Print and shaded views of the part. All mm, measured from the part's lowest x, y and z. Round coordinates to 2 decimals unless told otherwise and drop trailing zeros. Order: outer loops, then holes, each group sorted by start corner. A loop starts at its lowest first (then second) coordinate and runs counter-clockwise, first axis right, second up. Notation, with made-up numbers: (-20.5, 55) -> (34.5, 55) arc R29 cw to (34.5, 86) -> close; hole circle Ø4 at (10.25, -1). An arc over 180 degrees is marked (long way). Answer as CSV lines item,"result".
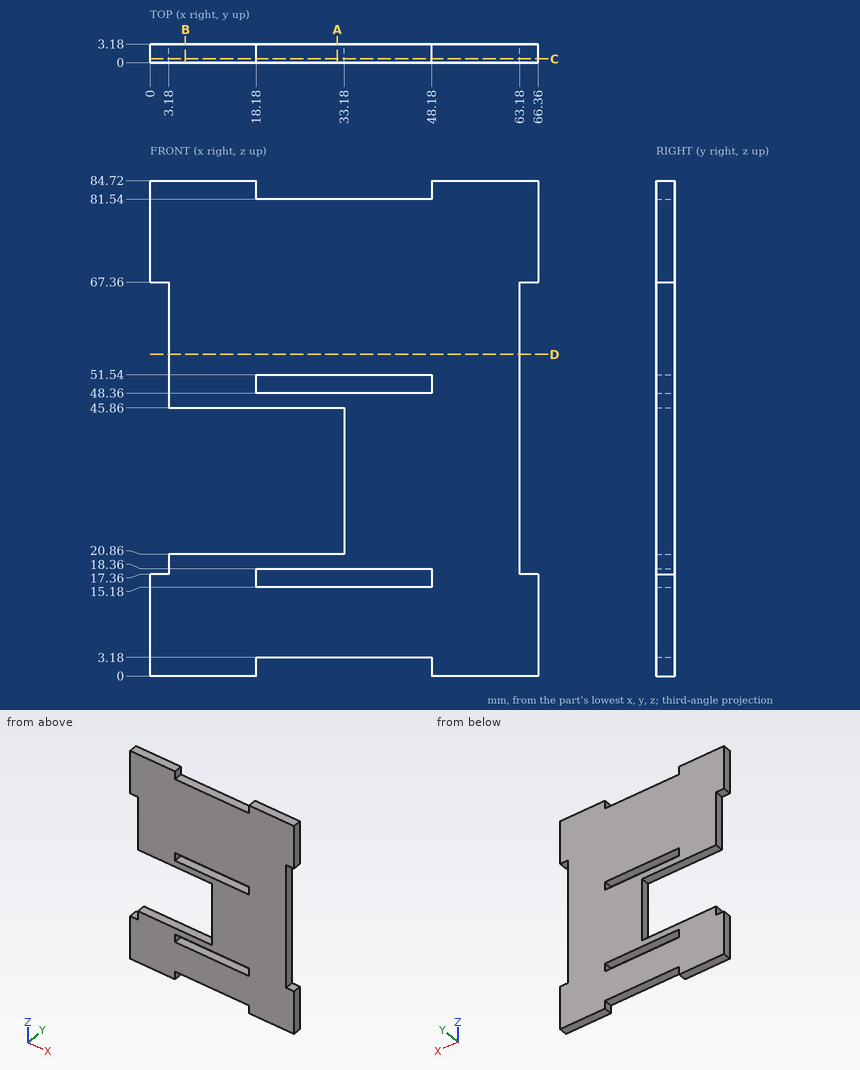
Q1. Saw through at C-C (y = 0.65). State how many separate pieces and enclosed holes the cut face has, plus the area to 3 significant figures.
Checks:
separate pieces,"1"
enclosed holes,"2"
area,"4,170 mm²"
Q2. Flat gauge pins, fed straight in: pin 1 (1.5 mm diameter, centred on y = 2, z = 48, fed in from -X); pin 2 (1.6 mm diameter, centred on x = 33, y = 1, fed in from -Z); pin 3 (1.6 mm diameter, centred on x = 20, y = 2, fed in from +Z). Where does each tip first touch, or does it go through?
Checks:
pin 1,"x = 3.18"
pin 2,"z = 3.18"
pin 3,"z = 81.54"
Q3. Saw through at A-A (x = 32). Write the cut outline in (y, z).
Checks:
outline,"(0, 3.18) -> (3.18, 3.18) -> (3.18, 15.18) -> (0, 15.18) -> close; (0, 18.36) -> (3.18, 18.36) -> (3.18, 20.86) -> (0, 20.86) -> close; (0, 45.86) -> (3.18, 45.86) -> (3.18, 48.36) -> (0, 48.36) -> close; (0, 51.54) -> (3.18, 51.54) -> (3.18, 81.54) -> (0, 81.54) -> close"
Q4. Wall check: L1, parallel to Z at x = 34, y = 1.9; L2, parallel to Z at x = 25, y = 1.1; L3, parallel to Z at x = 8, y = 2.25. Give the ranges that are in metal, low to high. Write a range as [from, to].
Checks:
L1,"[3.18, 15.18], [18.36, 48.36], [51.54, 81.54]"
L2,"[3.18, 15.18], [18.36, 20.86], [45.86, 48.36], [51.54, 81.54]"
L3,"[0, 20.86], [45.86, 84.72]"
Q5. Saw through at B-B (x = 6). Write the cut outline in (y, z).
Checks:
outline,"(0, 0) -> (3.18, 0) -> (3.18, 20.86) -> (0, 20.86) -> close; (0, 45.86) -> (3.18, 45.86) -> (3.18, 84.72) -> (0, 84.72) -> close"
Q6. Saw through at D-D (z = 55). Write the cut outline in (x, y).
Checks:
outline,"(3.18, 0) -> (63.18, 0) -> (63.18, 3.18) -> (3.18, 3.18) -> close"
